```python
from build123d import *

# Parameters (mm, degrees)
BOSS_EXTRUDE1_DEPTH     = 450
SKETCH2_R               = 1.75
CUT_EXTRUDE1_DEPTH      = 10
SKETCH3_R               = 3
CUT_EXTRUDE2_DEPTH      = 4
CHAMFER1_SIZE           = 0.5
CHAMFER1_SIZE2          = 1.743707222
CHAMFER1_PART_2_SIZE    = 0.5
CHAMFER1_PART_2_SIZE2   = 1.743707222
FILLET1_R               = 0.5
SKETCH4_W               = 45
SKETCH4_H               = 180.260452365
SKETCH4_H_2             = 288.291106743
CUT_EXTRUDE3_DEPTH      = 1
CUT_EXTRUDE3_DEPTH_BACK = 9


with BuildPart() as part:
    # Sketch1 → Boss-Extrude1 (new body)
    with BuildSketch(Plane(origin=(0, 0, 0), x_dir=(0, 0, -1), z_dir=(1, 0, 0))):
        Polygon((-0.5, 6), (4, 6), (4, -6), (-0.5, -6), (-0.5, -4.25), (-2.5, -4.25), (-2.5, -6), (-4, -6), (-4, 6), (-2.5, 6), (-2.5, 4.25), (-0.5, 4.25), align=None)
    extrude(amount=BOSS_EXTRUDE1_DEPTH)

    # Sketch2 → Cut-Extrude1 (cut)
    with BuildSketch(Plane.XY.offset(4)):
        with Locations((13, 0)):
            Circle(SKETCH2_R)
        with Locations((38, 0)):
            Circle(SKETCH2_R)
        with Locations((63, 0)):
            Circle(SKETCH2_R)
        with Locations((88, 0)):
            Circle(SKETCH2_R)
        with Locations((113, 0)):
            Circle(SKETCH2_R)
        with Locations((138, 0)):
            Circle(SKETCH2_R)
        with Locations((163, 0)):
            Circle(SKETCH2_R)
        with Locations((188, 0)):
            Circle(SKETCH2_R)
        with Locations((213, 0)):
            Circle(SKETCH2_R)
        with Locations((238, 0)):
            Circle(SKETCH2_R)
        with Locations((263, 0)):
            Circle(SKETCH2_R)
        with Locations((288, 0)):
            Circle(SKETCH2_R)
        with Locations((313, 0)):
            Circle(SKETCH2_R)
        with Locations((338, 0)):
            Circle(SKETCH2_R)
        with Locations((363, 0)):
            Circle(SKETCH2_R)
        with Locations((388, 0)):
            Circle(SKETCH2_R)
        with Locations((413, 0)):
            Circle(SKETCH2_R)
        with Locations((438, 0)):
            Circle(SKETCH2_R)
    extrude(amount=-CUT_EXTRUDE1_DEPTH, mode=Mode.SUBTRACT)

    # Sketch3 → Cut-Extrude2 (cut)
    with BuildSketch(Plane.XY.offset(4)):
        with Locations((13, 0)):
            Circle(SKETCH3_R)
        with Locations((38, 0)):
            Circle(SKETCH3_R)
        with Locations((63, 0)):
            Circle(SKETCH3_R)
        with Locations((88, 0)):
            Circle(SKETCH3_R)
        with Locations((113, 0)):
            Circle(SKETCH3_R)
        with Locations((138, 0)):
            Circle(SKETCH3_R)
        with Locations((163, 0)):
            Circle(SKETCH3_R)
        with Locations((188, 0)):
            Circle(SKETCH3_R)
        with Locations((213, 0)):
            Circle(SKETCH3_R)
        with Locations((238, 0)):
            Circle(SKETCH3_R)
        with Locations((263, 0)):
            Circle(SKETCH3_R)
        with Locations((288, 0)):
            Circle(SKETCH3_R)
        with Locations((313, 0)):
            Circle(SKETCH3_R)
        with Locations((338, 0)):
            Circle(SKETCH3_R)
        with Locations((363, 0)):
            Circle(SKETCH3_R)
        with Locations((388, 0)):
            Circle(SKETCH3_R)
        with Locations((413, 0)):
            Circle(SKETCH3_R)
        with Locations((438, 0)):
            Circle(SKETCH3_R)
    extrude(amount=-CUT_EXTRUDE2_DEPTH, mode=Mode.SUBTRACT)

    # Chamfer1
    chamfer1_edges = [part.edges().sort_by_distance(p)[0] for p in [
        (225, -4.25, 0.5),
        (225, -4.25, 2.5),
    ]]
    chamfer1_side = [part.faces().sort_by_distance(p)[0] for p in [
        (225, -4.25, 1.5),
    ]]
    chamfer(chamfer1_edges, length=CHAMFER1_SIZE, length2=CHAMFER1_SIZE2, reference=chamfer1_side[0])

    # Chamfer1 part 2
    chamfer1_part_2_edges = [part.edges().sort_by_distance(p)[0] for p in [
        (225, 4.25, 2.5),
        (225, 4.25, 0.5),
    ]]
    chamfer1_part_2_side = [part.faces().sort_by_distance(p)[0] for p in [
        (225, 4.25, 1.5),
    ]]
    chamfer(chamfer1_part_2_edges, length=CHAMFER1_PART_2_SIZE, length2=CHAMFER1_PART_2_SIZE2, reference=chamfer1_part_2_side[0])

    # Fillet1
    fillet1_edges = [part.edges().sort_by_distance(p)[0] for p in [
        (450, -6, -1.75),
        (450, 0, -4),
        (450, 6, -1.75),
        (450, 6, 3.25),
        (450, 0, 4),
        (450, -6, 3.25),
        (0, -6, 3.25),
        (0, -6, -1.75),
        (0, 0, -4),
        (0, 6, -1.75),
        (0, 6, 3.25),
        (0, 0, 4),
        (225, -4.25, 1),
        (225, -4.25, 2),
        (225, 4.25, 2),
        (225, 4.25, 1),
        (225, -6, 4),
        (225, 6, 4),
        (225, -6, -4),
        (225, 6, -4),
    ]]
    fillet(fillet1_edges, radius=FILLET1_R)

    # Sketch4 → Cut-Extrude3 (cut, two sides)
    with BuildSketch(Plane.XY.offset(4)) as cut_extrude3_sk:
        with Locations((22.5, -21.668939395)):
            Rectangle(SKETCH4_W, SKETCH4_H)
        with Locations((427.5, 22.925109796)):
            Rectangle(SKETCH4_W, SKETCH4_H_2)
    extrude(amount=CUT_EXTRUDE3_DEPTH, mode=Mode.SUBTRACT)
    extrude(cut_extrude3_sk.sketch, amount=-CUT_EXTRUDE3_DEPTH_BACK, mode=Mode.SUBTRACT)


solid = part.part
```
Verification items for the finished model (mm, model axes). A direction names the side the tool comes from. Give positions to 0.01 mm unless a question says otherwise; leave off trailing zeros. Return JSON: item names as keys, results as strings. Group by question number.
1) Mould release check, pull along X, two halves, no side actions. Record for faces 1 (the face through (222, 0, 4)), 2 (the face through (45, 0, 0)), 3 (the face through (285, 0, 2)): pulls with the +X half, pulls with the -X half, needs draft (parallel to the pull), parting line crosses it, or undercut.
2) Go/stop test with flat-tipped pins: pin 1 Ø3 at (x, y) = (188, 0) entering from -Z; pin 2 Ø3 at (x, y) = (388.5, 0.5) entering from +Z. Record where each tip stops, or that it passes through.
3) Access from +Z, -Z, +X, -X, +Y, -Y to the whole of each face (thin tool, end or side, straight path). Record for faces 4 (the face through (405, 0, 0)), 5 (the face through (85, 0, 2)).
4) Scan lines: line 1 (Z direction, x = 326, y = -4.75); line 2 (Y direction, x = 188, z = -1.7); line 3 (Z direction, x = 138, y = -2.75). Record each from-to range of solid material in increasing order.
5) Section check A-A on z = -1.5. Give the number of separate pieces and of enclosed holes in the cut face, and give its area (3 significant figures).
Answer block:
{
 "1": {"face 1": "needs draft", "face 2": "pulls with the -X half", "face 3": "undercut"},
 "2": {"pin 1": "passes through", "pin 2": "stops at z = 0"},
 "3": {"face 4": "+Z, -Z, +X, +Y, -Y", "face 5": "+Z"},
 "4": {"line 1": "z = -4 to 0.86, 2.14 to 4", "line 2": "y = -6 to -1.75, 1.75 to 6", "line 3": "z = -4 to 0"},
 "5": {"separate pieces": "1", "enclosed holes": "14", "area": "4,190 mm^2"}
}
